The listing builds one solid part. Answer for the finished solid, in the listing's coordinates (mm). Round coordinates to 2 decimals unless told otherwise and drop trailing zeros. Order: outer loops, then holes, each group sorted by start corner. A loop starts at its lowest first (then second) coordinate and runs counter-clockwise, first axis right, second up. Notation, with made-up numbers: (34, 65) -> (51, 65) arc R23 ccw to (51, 81) -> close; hole circle Ø8 at (40.5, 37.25). An arc over 180 degrees is marked (long way). Return JSON: item names as keys, results as strings. Group by question number.
(1) The part is cut by section A-A (x = 133.5). Count the separate pieces of the cut face and the enclosed holes in it, plus the area to 3 significant figures.
(2) The part is cut by section B-B (z = -100). Determine the outline of the cut face in (x, y).
(3) The part is cut by section C-C (x = 9.5). Determine the outline of the cut face in (y, z).
(4) Each of these flat-tipped pins is pushed along its axis until it touches: pin 1 (0.5 mm diameter, centred on y = -58.5, z = -0.5, fed in from -X); pin 2 (0.5 mm diameter, centred on x = 127, y = -58.5, fed in from -Z); pin 3 (0.5 mm diameter, centred on y = -58.5, z = -184, fed in from +X). Where does it stop, or does it pass through?
(5) Consider line 1 (X direction, y = -58.4, z = -101); line 2 (X direction, y = -58.55, z = -165); line 3 (Z direction, x = 34, y = -58.4). Determine where each line is inside the solid, lowest interval first. Write a range as [from, to].
from build123d import *

# Parameters (mm, degrees)
EXTRUDE_1_DEPTH     = 0.5
EXTRUDE_2_DEPTH     = 104.5
SKETCH_8_W          = 60
SKETCH_8_H          = 8
SKETCH_8_W_2        = 60.000005443
CUT_EXTRUDE_2_DEPTH = 10
EXTRUDE_4_DEPTH     = 2.5
SKETCH_7_R          = 3.5
SKETCH_7_R_2        = 0.5
CUT_EXTRUDE_4_DEPTH = 244
SKETCH_10_W         = 3
SKETCH_10_H         = 95.004122321
SKETCH_10_H_2       = 102.964943566
CUT_EXTRUDE_5_DEPTH = 284
SKETCH_11_W         = 204
SKETCH_11_H         = 57
CUT_EXTRUDE_6_DEPTH = 284
SKETCH_13_W         = 2.47
SKETCH_13_H         = 15
CUT_EXTRUDE_7_DEPTH = 284
SKETCH_14_W         = 15
SKETCH_14_H         = 3
EXTRUDE_5_DEPTH     = 1


with BuildPart() as part:
    # Sketch 1 → Extrude 1 (new body)
    with BuildSketch(Plane.XY):
        Polygon((0, -1.078212291), (0, -59.078212291), (150, -59.078212291), (150, -56.078212291), (24.720670391, -21.433997855), (24.720670391, -1.078212291), align=None)
    extrude(amount=EXTRUDE_1_DEPTH)

    # Sketch 2 → Extrude 2 (add)
    with BuildSketch(Plane(origin=(0, 0, 0), x_dir=(-1, 0, 0), z_dir=(0, 0, -1))):
        with BuildLine():
            Line((-2.47, -1.078212291), (-2.47, -58.078212291))
            Line((-2.47, -58.078212291), (-149, -58.078212291))
            ThreePointArc((-149, -58.078212291), (-149.5, -58.578212291), (-149, -59.078212291))
            Line((-149, -59.078212291), (0, -59.078212291))
            Line((0, -59.078212291), (0, -1.078212291))
            Line((0, -1.078212291), (-2.47, -1.078212291))
        make_face()
    extrude(amount=EXTRUDE_2_DEPTH)

    # Mirror 3: part across plane


with BuildPart() as part_1:
    add(part.part)
    add(part.part.mirror(Plane(origin=(149, -58.578212291, -104.5), x_dir=(1, 0, 0), z_dir=(0, 0, -1))))

    # Sketch 8 → Cut-Extrude 2 (cut)
    with BuildSketch(Plane(origin=(0, -58.078212291, 0), x_dir=(1, 0, 0), z_dir=(0, 1, 0))):
        with Locations((121.473716686, 5)):
            Rectangle(SKETCH_8_W, SKETCH_8_H)
        with Locations((121.473713965, 15)):
            Rectangle(SKETCH_8_W_2, SKETCH_8_H)
        with Locations((121.473713965, 24.421052632)):
            Rectangle(SKETCH_8_W_2, SKETCH_8_H)
        with Locations((121.473713965, 33.842105263)):
            Rectangle(SKETCH_8_W_2, SKETCH_8_H)
        with Locations((121.473713965, 43.263157895)):
            Rectangle(SKETCH_8_W_2, SKETCH_8_H)
        with Locations((121.473713965, 52.684210526)):
            Rectangle(SKETCH_8_W_2, SKETCH_8_H)
        with Locations((121.473713965, 62.105263158)):
            Rectangle(SKETCH_8_W_2, SKETCH_8_H)
        with Locations((121.473713965, 71.526315789)):
            Rectangle(SKETCH_8_W_2, SKETCH_8_H)
        with Locations((121.473713965, 80.947368421)):
            Rectangle(SKETCH_8_W_2, SKETCH_8_H)
        with Locations((121.473713965, 90.368421053)):
            Rectangle(SKETCH_8_W_2, SKETCH_8_H)
        with Locations((121.473713965, 99.789473684)):
            Rectangle(SKETCH_8_W_2, SKETCH_8_H)
        with Locations((121.473713965, 109.210526316)):
            Rectangle(SKETCH_8_W_2, SKETCH_8_H)
        with Locations((121.473713965, 118.631578947)):
            Rectangle(SKETCH_8_W_2, SKETCH_8_H)
        with Locations((121.473713965, 128.052631579)):
            Rectangle(SKETCH_8_W_2, SKETCH_8_H)
        with Locations((121.473713965, 137.473684211)):
            Rectangle(SKETCH_8_W_2, SKETCH_8_H)
        with Locations((121.473713965, 146.894736842)):
            Rectangle(SKETCH_8_W_2, SKETCH_8_H)
        with Locations((121.473713965, 156.315789474)):
            Rectangle(SKETCH_8_W_2, SKETCH_8_H)
        with Locations((121.473713965, 165.736842105)):
            Rectangle(SKETCH_8_W_2, SKETCH_8_H)
        with Locations((121.473713965, 175.157894737)):
            Rectangle(SKETCH_8_W_2, SKETCH_8_H)
        with Locations((121.473713965, 184.578947368)):
            Rectangle(SKETCH_8_W_2, SKETCH_8_H)
        with Locations((121.473713965, 194)):
            Rectangle(SKETCH_8_W_2, SKETCH_8_H)
        with Locations((121.473716686, 204)):
            Rectangle(SKETCH_8_W, SKETCH_8_H)
    extrude(amount=-CUT_EXTRUDE_2_DEPTH, mode=Mode.SUBTRACT)

    # Sketch 1_3 → Extrude 4 (add)
    with BuildSketch(Plane.XY):
        Polygon((0, -1.078212291), (0, -59.078212291), (150, -59.078212291), (150, -56.078212291), (24.720670391, -21.433997855), (24.720670391, -1.078212291), align=None)
    extrude_4 = extrude(amount=-EXTRUDE_4_DEPTH)

    # Mirror 4: Extrude 4 across plane
    add(extrude_4.mirror(Plane.XY.offset(-104.5)))

    # Mirror 5: Extrude 4 across plane
    add(extrude_4.mirror(Plane.XY.offset(-104.5)))

    # Sketch 7 → Cut-Extrude 4 (cut)
    with BuildSketch(Plane.XY.offset(0.5)):
        with Locations(Location((8, -45.078212291, 0), (0, 0, 180))):
            Circle(SKETCH_7_R)
        with Locations(Location((25, -45.078212291, 0), (0, 0, 180))):
            Circle(SKETCH_7_R_2)
        with Locations(Location((23, -45.078212291, 0), (0, 0, 180))):
            Circle(SKETCH_7_R_2)
    extrude(amount=-CUT_EXTRUDE_4_DEPTH, mode=Mode.SUBTRACT)

    # Sketch 10 → Cut-Extrude 5 (cut)
    with BuildSketch(Plane(origin=(150, 0, 0), x_dir=(0, 0, -1), z_dir=(1, 0, 0))):
        with Locations((1, -11.576151131)):
            Rectangle(SKETCH_10_W, SKETCH_10_H)
        with Locations((208, -7.595740508)):
            Rectangle(SKETCH_10_W, SKETCH_10_H_2)
    extrude(amount=-CUT_EXTRUDE_5_DEPTH, mode=Mode.SUBTRACT)

    # Sketch 11 → Cut-Extrude 6 (cut)
    with BuildSketch(Plane(origin=(2.47, 0, 0), x_dir=(0, 0, -1), z_dir=(1, 0, 0))):
        with Locations((104.5, -29.578212291)):
            Rectangle(SKETCH_11_W, SKETCH_11_H)
    extrude(amount=-CUT_EXTRUDE_6_DEPTH, mode=Mode.SUBTRACT)

    # Sketch 13 → Cut-Extrude 7 (cut)
    with BuildSketch(Plane(origin=(0, -58.078212291, 0), x_dir=(1, 0, 0), z_dir=(0, 1, 0))):
        with Locations((1.235, 40)):
            Rectangle(SKETCH_13_W, SKETCH_13_H)
        with Locations((1.235, 169)):
            Rectangle(SKETCH_13_W, SKETCH_13_H)
    extrude(amount=-CUT_EXTRUDE_7_DEPTH, mode=Mode.SUBTRACT)

    # Sketch 14 → Extrude 5 (add)
    with BuildSketch(Plane(origin=(0, -59.078212291, 0), x_dir=(-1, 0, 0), z_dir=(0, -1, 0))):
        with Locations((-83.973716686, 1)):
            Rectangle(SKETCH_14_W, SKETCH_14_H)
        with Locations((-53.973716686, 1)):
            Rectangle(SKETCH_14_W, SKETCH_14_H)
    extrude_5 = extrude(amount=-EXTRUDE_5_DEPTH)

    # Mirror 6: Extrude 5 across plane
    add(extrude_5.mirror(Plane.XY.offset(-104.5)))


solid = part_1.part
Answer below:
{
 "1": {"separate pieces": "21", "enclosed holes": "0", "area": "31.0 mm²"},
 "2": {"outline": "(0, -59.08) -> (91.47, -59.08) -> (91.47, -58.08) -> (0, -58.08) -> close"},
 "3": {"outline": "(-59.08, -206.5) -> (-58.08, -206.5) -> (-58.08, -2.5) -> (-59.08, -2.5) -> close"},
 "4": {"pin 1": "stops at x = 46.47", "pin 2": "stops at z = -200", "pin 3": "stops at x = 91.47"},
 "5": {"line 1": "x = [0, 91.47]", "line 2": "x = [2.47, 91.47]", "line 3": "z = [-206.5, -2.5]"}
}
